from build123d import *

# Parameters (mm, degrees)
SKETCH3_R          = 19.05
SKETCH3_R_2        = 9.525
SKETCH3_R_3        = 18.988330579
CUT_EXTRUDE2_DEPTH = 146.863175777


with BuildPart() as part:
    # Sketch1 → Revolve1 (revolve)
    with BuildSketch(Plane.XY, mode=Mode.PRIVATE) as revolve1_sk:
        Polygon((0, 0), (101.558930414, 0), (101.558930414, 7.658156006), (94.018592193, 7.658156006), (94.018592193, 17.79048549), (101.558930414, 17.79048549), (101.558930414, 25.448641496), (0, 25.448641496), align=None)
    revolve(revolve1_sk.sketch.rotate(Axis((0, 25.448641496, 0), (0, -1, 0)), 90), axis=Axis((0, 25.448641496, 0), (0, -1, 0)))

    # Sketch3 → Cut-Extrude2 (cut, through all)
    with BuildSketch(Plane(origin=(0, 25.448641496, 0), x_dir=(1, 0, 0), z_dir=(0, 1, 0))):
        with BuildLine():
            Line((3.175, 10.580896572), (-3.175, 10.580896572))
            Line((-3.175, 10.580896572), (-3.175, 5.499261314))
            ThreePointArc((-3.175, 5.499261314), (0, -6.35), (3.175, 5.499261314))
            Line((3.175, 5.499261314), (3.175, 10.580896572))
        make_face()
        with Locations(Location((63.5, 0, 0), (0, 0, 270))):
            Circle(SKETCH3_R)
        with Locations(Location((47.997207269, 41.575450622, 0), (0, 0, 270))):
            Circle(SKETCH3_R_2)
        with Locations(Location((46.521487533, -43.220379426, 0), (0, 0, 270))):
            Circle(SKETCH3_R_2)
        with Locations(Location((0, 63.5, 0), (0, 0, 270))):
            Circle(SKETCH3_R)
        with Locations(Location((0, -63.5, 0), (0, 0, 270))):
            Circle(SKETCH3_R)
        with Locations(Location((-47.659859298, 41.961742239, 0), (0, 0, 270))):
            Circle(SKETCH3_R_2)
        with Locations(Location((-44.386705472, -45.410025075, 0), (0, 0, 270))):
            Circle(SKETCH3_R_2)
        with Locations(Location((-63.5, 0, 0), (0, 0, 270))):
            Circle(SKETCH3_R_3)
    extrude(amount=-CUT_EXTRUDE2_DEPTH, mode=Mode.SUBTRACT)


solid = part.part
The listing builds one solid part. Answer for the finished solid, in the listing's coordinates (mm). A direction names the side the tool comes from. Coordinates: 2 decimals unless noted, no trailing zeros. Loops run counter-clockwise (first coordinate to the right, second up) from the corner with the lowest first, then second, coordinate; pieces in that order, holes last. Notation, with made-up numbers: (-8.5, -36) -> (32.5, -36) arc R13 cw to (32.5, -28) -> close; hole circle Ø9 at (77.25, 31). An arc over 180 degrees is marked (long way). Write item = value, one per line. Start each with the question number.
1) The mould has two halves that part along Z. Classify faces 4 (the face through (-68.64, 21.67, -74.85)), 5 (the face through (30, 17.79, -90)), 6 (the face through (3.175, 13, -8)): released by +Z, released by -Z, zero draft, split by the parting line, or undercut.
2) A tool of negligible diameter and unlimited length cuts with its end or side. For faces 1 (the face through (-3.175, 13, -8)), 2 (the face through (-1, 0, -21)), 3 (the face through (90, 7.658, 30)), from which of +Z, -Z, +X, -X, +Y, -Y can it reach the whole face along a straight path? Write none if from no direction.
3) A cutting plane is placed at C-C (x = 63.5). Give the vertices of the cut face in (y, z), then the cut area to 3 significant figures.
4) Straight lines are drawn through the part: line 1 (X direction, y = 9.5, z = 48.5); line 2 (X direction, y = 18.25, z = -35); line 3 (Z direction, x = -2.5, y = 20.25). For each, find the intervals that lie inside material, in ascending order. Write a range as from..to.
5) A cutting plane is placed at A-A (z = 0). Give the vertices of the cut face in (x, y).
6) A cutting plane is placed at D-D (y = 12). Count the separate pieces of the cut face and the enclosed holes in it, then the cut area to 3 significant figures.
7) A cutting plane is placed at B-B (x = 0). Give the vertices of the cut face in (y, z), then the cut area to 3 significant figures.
8) Given pin 1 Ø11.5 at (x, z) = (-47.66, -41.96) entering from +Y; pin 2 Ø5 at (y, z) = (19.5, -59.5) entering from -X; pin 3 Ø5 at (x, y) = (-37, 4.5) entering from -Z; pin 4 Ø8 at (x, y) = (33, 4.5) entering from +Z, each flat-ended and moving along its own axis, determine where each tip first touches the part or whether it passes through.
Responses:
q1.face_4 = split by the parting line
q1.face_5 = zero draft
q1.face_6 = undercut
q2.face_1 = +Y, -Y
q2.face_2 = +Z, -Z, +X, -X, -Y
q2.face_3 = none
q3.outline = (0, -79.26) -> (7.66, -79.26) -> (7.66, -69.33) -> (17.79, -69.33) -> (17.79, -79.26) -> (25.45, -79.26) -> (25.45, -19.05) -> (0, -19.05) -> close; (0, 19.05) -> (25.45, 19.05) -> (25.45, 79.26) -> (17.79, 79.26) -> (17.79, 69.33) -> (7.66, 69.33) -> (7.66, 79.26) -> (0, 79.26) -> close
q3.area = 2,860 mm²
q4.line_1 = -80.54..-53.4, -35.38..-11.74, 11.74..38.59, 54.45..80.54
q4.line_2 = -95.34..-54.16, -41.16..41.11, 54.89..95.34
q4.line_3 = -101.53..-82.39, -44.61..-10.58, 5.84..44.61, 82.39..101.53
q5.outline = (-101.56, 0) -> (-82.49, 0) -> (-82.49, 25.45) -> (-101.56, 25.45) -> (-101.56, 17.79) -> (-94.02, 17.79) -> (-94.02, 7.66) -> (-101.56, 7.66) -> close; (-44.51, 0) -> (-6.35, 0) -> (-6.35, 25.45) -> (-44.51, 25.45) -> close; (6.35, 0) -> (44.45, 0) -> (44.45, 25.45) -> (6.35, 25.45) -> close; (82.55, 0) -> (101.56, 0) -> (101.56, 7.66) -> (94.02, 7.66) -> (94.02, 17.79) -> (101.56, 17.79) -> (101.56, 25.45) -> (82.55, 25.45) -> close
q6.separate_pieces = 1
q6.enclosed_holes = 9
q6.area = 21,900 mm²
q7.outline = (0, -101.56) -> (7.66, -101.56) -> (7.66, -94.02) -> (17.79, -94.02) -> (17.79, -101.56) -> (25.45, -101.56) -> (25.45, -82.55) -> (0, -82.55) -> close; (0, -44.45) -> (25.45, -44.45) -> (25.45, -10.58) -> (0, -10.58) -> close; (0, 6.35) -> (25.45, 6.35) -> (25.45, 44.45) -> (0, 44.45) -> close; (0, 82.55) -> (25.45, 82.55) -> (25.45, 101.56) -> (17.79, 101.56) -> (17.79, 94.02) -> (7.66, 94.02) -> (7.66, 101.56) -> (0, 101.56) -> close
q7.area = 2,650 mm²
q8.pin_1 = through
q8.pin_2 = -84.05
q8.pin_3 = -95.52
q8.pin_4 = 97.33
